```python
from build123d import *

# Parameters (mm, degrees)
SKETCH1_R           = 67
SKETCH1_R_2         = 25
BOSS_EXTRUDE1_DEPTH = 15
SKETCH2_R           = 100
SKETCH2_R_2         = 25
BOSS_EXTRUDE2_DEPTH = 15
SKETCH4_R           = 4
CUT_EXTRUDE2_DEPTH  = 15
CIRPATTERN1_COUNT   = 8


with BuildPart() as part:
    # Sketch1 → Boss-Extrude1 (new body)
    with BuildSketch(Plane(origin=(0, 0, 0), x_dir=(1, 0, 0), z_dir=(0, 1, 0))):
        with Locations(Location((0, 0, 0), (0, 0, 270))):
            Circle(SKETCH1_R)
        with Locations(Location((-33.5, 0, 0), (0, 0, 270))):
            Circle(SKETCH1_R_2, mode=Mode.SUBTRACT)
        with Locations(Location((33.5, 0, 0), (0, 0, 270))):
            Circle(SKETCH1_R_2, mode=Mode.SUBTRACT)
    extrude(amount=BOSS_EXTRUDE1_DEPTH)

    # Sketch2 → Boss-Extrude2 (add)
    with BuildSketch(Plane(origin=(0, 15, 0), x_dir=(1, 0, 0), z_dir=(0, 1, 0))):
        with Locations(Location((0, 0, 0), (0, 0, 270))):
            Circle(SKETCH2_R)
        with Locations(Location((33.5, 0, 0), (0, 0, 270))):
            Circle(SKETCH2_R_2, mode=Mode.SUBTRACT)
        with Locations(Location((-33.5, 0, 0), (0, 0, 270))):
            Circle(SKETCH2_R_2, mode=Mode.SUBTRACT)
    extrude(amount=BOSS_EXTRUDE2_DEPTH)

    # Sketch4 → Cut-Extrude2 (cut)
    with BuildSketch(Plane(origin=(0, 30, 0), x_dir=(1, 0, 0), z_dir=(0, 1, 0))):
        with Locations(Location((-92, 0, 0), (0, 0, 270))):
            Circle(SKETCH4_R)
    cut_extrude2 = extrude(amount=-CUT_EXTRUDE2_DEPTH, mode=Mode.SUBTRACT)

    # CirPattern1: Cut-Extrude2 ×8 about axis
    cirpattern1_axis = Axis((0, 0, 0), (0, 1, 0))
    for i in range(1, CIRPATTERN1_COUNT):
        add(cut_extrude2.rotate(cirpattern1_axis, i * 360 / CIRPATTERN1_COUNT), mode=Mode.SUBTRACT)


solid = part.part
```
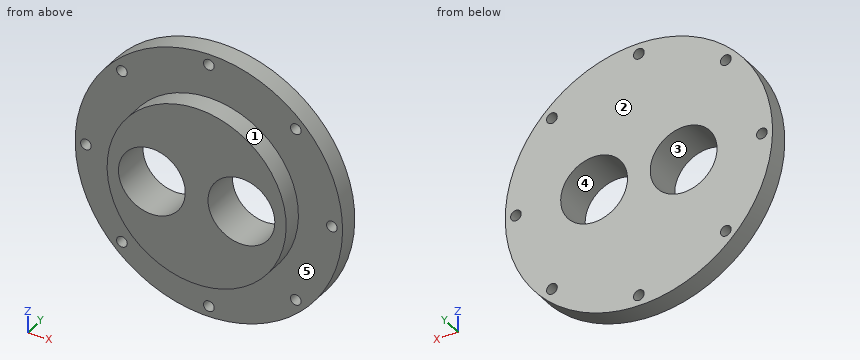
Source: CAD feature listing. Evaluate the final solid. Frame: model axes, mm. Face numbers are marked on the shaded views. A direction names the side the tool comes from. Round coordinates to 2 decimals unless told otherwise and drop trailing zeros. Loops run counter-clockwise (first coordinate to the right, second up) from the corner with the lowest first, then second, coordinate; pieces in that order, holes last.
(1) Section query D-D (y = 2.75). Output: boundary loops of the cut face in (x, z), and give its area (3 significant figures).
From the geometry:
outline: circle Ø134 at (0, 0); hole circle Ø50 at (-33.5, 0); hole circle Ø50 at (33.5, 0)
area: 10,200 mm2
(2) Pull-direction query (X, two-part tool) for the marked faces 1, 2 and 3; classes: +X half, -X half, draft (parallel to the pull), parting line (faces both ways), or undercut.
From the geometry:
face 1: parting line
face 2: draft
face 3: undercut
(3) Section query B-B (x = 0). Output: boundary loops of the cut face in (y, z).
From the geometry:
outline: (0, -67) - (15, -67) - (15, -88) - (30, -88) - (30, 88) - (15, 88) - (15, 67) - (0, 67) - close; (15, -100) - (30, -100) - (30, -96) - (15, -96) - close; (15, 96) - (30, 96) - (30, 100) - (15, 100) - close
(4) Access query for the marked faces 4 and 5. Directions: +Z, -Z, +X, -X, +Y, -Y. A direction counts if a zero-diameter tool reaches every point of the face in a straight line with its end or side. Return the directions, or none.
From the geometry:
face 4: +Y, -Y
face 5: -Y
(5) Contact query for flat-ended pins moving along their axis: pin 1 Ø13 at (x, z) = (0, -92) entering from -Y; pin 2 Ø10 at (y, z) = (14.5, 70.5) entering from -X; pin 3 Ø12 at (x, y) = (-64, 3.5) entering from -Z. Output: stop coordinate, or through.
From the geometry:
pin 1: stops at y = 15
pin 2: stops at x = -75.54
pin 3: stops at z = -33.54
(6) Material intervals for probe 1 along X at (y, z) = (17, 0); probe 2 along X at (y, z) = (17.5, -5.5); probe 3 along X at (y, z) = (21, 9.5), sorted ascending.
From the geometry:
probe 1: x = -100 to -96, -88 to -58.5, -8.5 to 8.5, 58.5 to 88, 96 to 100
probe 2: x = -99.85 to -57.89, -9.11 to 9.11, 57.89 to 99.85
probe 3: x = -99.55 to -56.62, -10.38 to 10.38, 56.62 to 99.55
(7) Section query C-C (x = 92). Output: boundary loops of the cut face in (y, z).
From the geometry:
outline: (15, -39.19) - (30, -39.19) - (30, -4) - (15, -4) - close; (15, 4) - (30, 4) - (30, 39.19) - (15, 39.19) - close
(8) Section query A-A (z = 0). Output: boundary loops of the cut face in (x, y).
From the geometry:
outline: (-100, 15) - (-96, 15) - (-96, 30) - (-100, 30) - close; (-88, 15) - (-67, 15) - (-67, 0) - (-58.5, 0) - (-58.5, 30) - (-88, 30) - close; (-8.5, 0) - (8.5, 0) - (8.5, 30) - (-8.5, 30) - close; (58.5, 0) - (67, 0) - (67, 15) - (88, 15) - (88, 30) - (58.5, 30) - close; (96, 15) - (100, 15) - (100, 30) - (96, 30) - close
